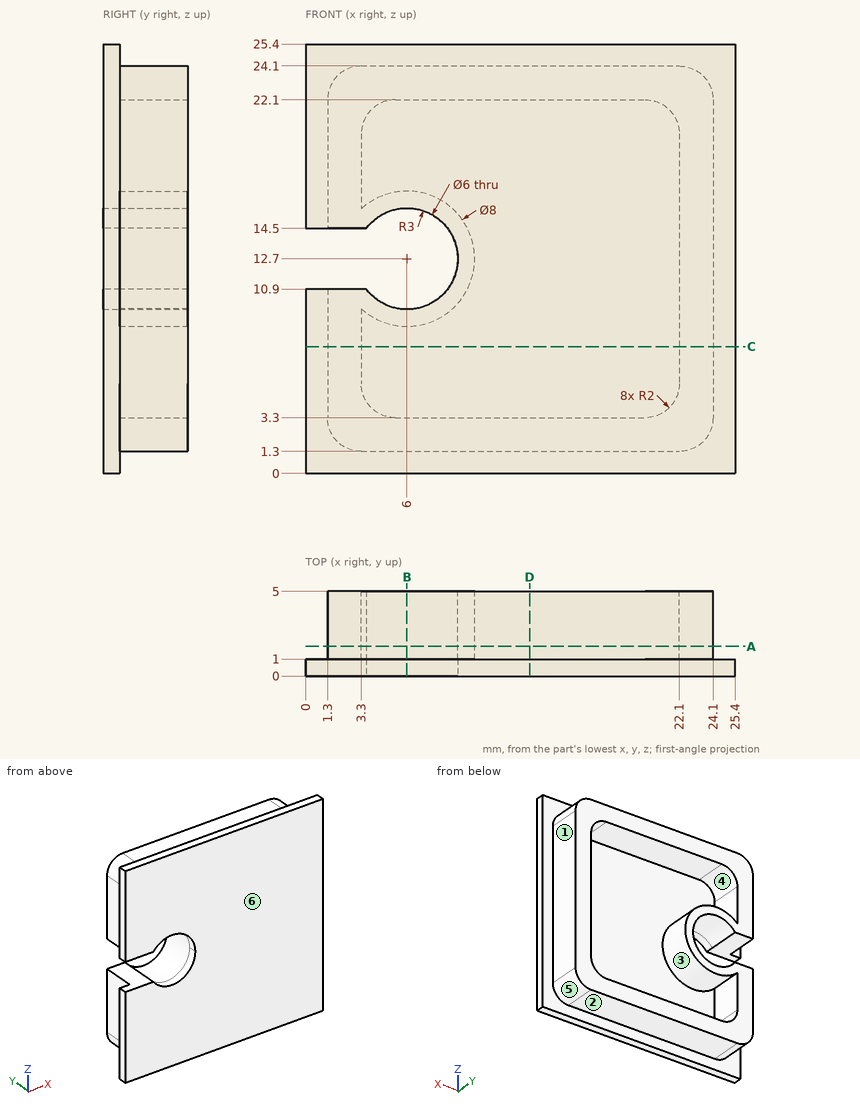
Could you check a few things on this drawing? It's one solid part, dimensions in mm from its lowest x, y, z. A direction names the side the tool comes from. Round coordinates to 2 decimals unless told otherwise and drop trailing zeros. Loops run counter-clockwise (first coordinate to the right, second up) from the corner with the lowest first, then second, coordinate; pieces in that order, holes last.
Q1. I want a section at C-C (z = 7.5). Write out the boundary of the cut face in (x, y), and give its area (3 significant figures).
Q2. On a 3-axis mill with a long thin cutter (end or side, diameter ignored), from which of +Z, -Z, +X, -X, +Y, -Y can I reach the whole of each face in a straight line? I mean the marked faces 4, 5 and 6. Say none if no direction works.
Q3. Thinking about a two-plate mould opening in Z: for the marked faces 1, 2 and 3, which applies, pulls with the +Z half, pulls with the -Z half, needs draft (parallel to the pull), parting line crosses it, or undercut?
Q4. For P1, Ø1.2, axis at x = 14.5, y = 4, coming from the +Z side; P2, Ø2, axis at y = 2.5, z = 14, coming from the -X side; P3, Ø3, axis at y = 3.5, z = 8.5, coming from the +X side; P4, Ø3.5, axis at x = 6, z = 12.7, coming from the +Y side, each with a flat end and sliding along its axis, tell me the tip position at first contact or that it passes through.
Q5. I want a section at A-A (y = 1.75). Write out the boundary of the cut face in (x, z).
Q6. I want a section at B-B (x = 6). Write out the boundary of the cut face in (y, z), and give its area (3 significant figures).
Q7. I want a section at D-D (x = 13.25). Write out the boundary of the cut face in (y, z).
Q8. Please list where these lines run through material, in increasing order: L1, parallel to Z at x = 6, y = 3.8; L2, parallel to Z at x = 20.25, y = 2.45; L3, parallel to X at y = 4.15, z = 12.7.
Answer below:
1. outline: (0, 0) - (25.4, 0) - (25.4, 1) - (24.1, 1) - (24.1, 5) - (22.1, 5) - (22.1, 1) - (3.3, 1) - (3.3, 5) - (1.3, 5) - (1.3, 1) - (0, 1) - close
1. area: 41.4 mm2
2. face 4: +Y
2. face 5: -Z, +X, +Y
2. face 6: +Z, -Z, +X, -X, -Y
3. face 1: needs draft
3. face 2: pulls with the -Z half
3. face 3: undercut
4. P1: stops at z = 24.1
4. P2: stops at x = 1.3
4. P3: stops at x = 24.1
4. P4: passes through
5. outline: (1.3, 3.3) arc R2 ccw to (3.3, 1.3) - (22.1, 1.3) arc R2 ccw to (24.1, 3.3) - (24.1, 22.1) arc R2 ccw to (22.1, 24.1) - (3.3, 24.1) arc R2 ccw to (1.3, 22.1) - (1.3, 14.5) - (3.6, 14.5) arc R3 cw (long way) to (3.6, 10.9) - (1.3, 10.9) - close; hole (3.3, 5.3) arc R2 ccw to (5.3, 3.3) - (20.1, 3.3) arc R2 ccw to (22.1, 5.3) - (22.1, 20.1) arc R2 ccw to (20.1, 22.1) - (5.3, 22.1) arc R2 ccw to (3.3, 20.1) - (3.3, 15.65) arc R4 cw (long way) to (3.3, 9.75) - close
6. outline: (0, 0) - (1, 0) - (1, 1.3) - (5, 1.3) - (5, 3.3) - (1, 3.3) - (1, 8.7) - (5, 8.7) - (5, 9.7) - (0, 9.7) - close; (0, 15.7) - (5, 15.7) - (5, 16.7) - (1, 16.7) - (1, 22.1) - (5, 22.1) - (5, 24.1) - (1, 24.1) - (1, 25.4) - (0, 25.4) - close
6. area: 43.4 mm2
7. outline: (0, 0) - (1, 0) - (1, 1.3) - (5, 1.3) - (5, 3.3) - (1, 3.3) - (1, 22.1) - (5, 22.1) - (5, 24.1) - (1, 24.1) - (1, 25.4) - (0, 25.4) - close
8. L1: z = 1.3 to 3.3, 8.7 to 9.7, 15.7 to 16.7, 22.1 to 24.1
8. L2: z = 1.3 to 3.31, 22.09 to 24.1
8. L3: x = 9 to 10, 22.1 to 24.1
